Part model, mm, in its own coordinate system. Face numbers are marked on the shaded views. A direction names the side the tool comes from. Coordinates: 2 decimals unless noted, no trailing zeros. Loops run counter-clockwise (first coordinate to the right, second up) from the corner with the lowest first, then second, coordinate; pieces in that order, holes last. Notation, with made-up numbers: (67, 49.25) -> (119, 49.25) arc R18 ccw to (119, 64.25) -> close; hole circle Ø3 at (-16.75, 71). An arc over 180 degrees is marked (long way). One line per item, written item: value. Start each with the question number.
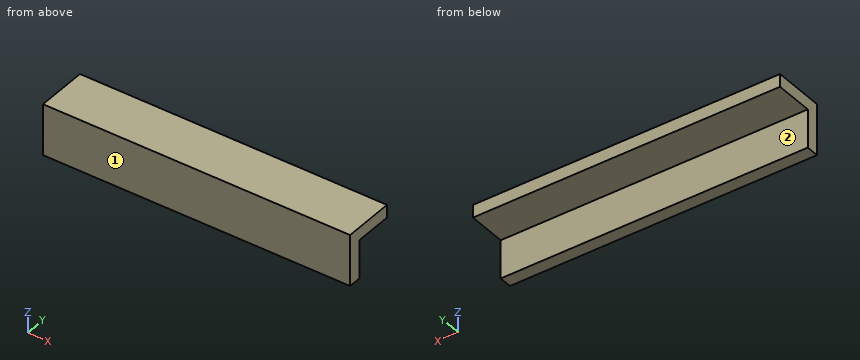
from build123d import *

# Parameters (mm, degrees)
SKETCH1_W           = 76.2
SKETCH1_H           = 12.7
BOSS_EXTRUDE1_DEPTH = 3.175
SKETCH7_W           = 76.2
SKETCH7_H           = 9.525
BOSS_EXTRUDE2_DEPTH = 3.175


with BuildPart() as part:
    # Sketch1 → Boss-Extrude1 (new body)
    with BuildSketch(Plane.XY):
        with Locations((33.686472643, 22.354273404)):
            Rectangle(SKETCH1_W, SKETCH1_H)
    extrude(amount=BOSS_EXTRUDE1_DEPTH)

    # Sketch7 → Boss-Extrude2 (add)
    with BuildSketch(Plane(origin=(0, 16.004273404, 0), x_dir=(-1, 0, 0), z_dir=(0, -1, 0))):
        with Locations((-33.686472643, 4.7625)):
            Rectangle(SKETCH7_W, SKETCH7_H)
    extrude(amount=-BOSS_EXTRUDE2_DEPTH)


solid = part.part
1) Slice it at A-A (x = 51.5). Give the cut face in (y, z) (3 decimals).
2) Tool access for the marked faces 1 and 2: list every direction of +Z, -Z, +X, -X, +Y, -Y with a clear straight run to the whole face (end or side of a thin tool).
3) Slice it at B-B (z = -5.25). Give the cut face in (x, y), then the cut area to 3 significant figures.
4) Probe line 1 (Y direction, x = 65, z = -0.25); line 2 (Z direction, x = 46, y = 22) (3 decimals). List the from-to ranges inside material, lowest first. Write a range as from..to.
5) Slice it at C-C (y = 25.25). Give the cut face in (x, z) (3 decimals), then the cut area to 3 significant figures.
6) Pin check, flat tips, straight feed: pin 1 Ø7.5 at (x, z) = (50, -5.5) entering from +Y; pin 2 Ø2 at (x, y) = (59, 21) entering from -Z. Stop position of each tip, or through.
Check sheet entries:
1. outline: (16.004, -9.525) -> (19.179, -9.525) -> (19.179, 0) -> (28.704, 0) -> (28.704, 3.175) -> (16.004, 3.175) -> close
2. face 1: +Z, -Z, +X, -X, -Y
2. face 2: -Z, +X, -X, +Y
3. outline: (-4.41, 16) -> (71.79, 16) -> (71.79, 19.18) -> (-4.41, 19.18) -> close
3. area: 242 mm^2
4. line 1: y = 16..19.18
4. line 2: z = 0..3.175
5. outline: (-4.414, 0) -> (71.786, 0) -> (71.786, 3.175) -> (-4.414, 3.175) -> close
5. area: 242 mm^2
6. pin 1: stops at y = 19.18
6. pin 2: stops at z = 0
